from build123d import *

# Parameters (mm, degrees)
SKETCH_1_R          = 14
EXTRUDE_1_DEPTH     = 2.5
SKETCH_2_R          = 1.45
EXTRUDE_2_DEPTH     = 1.5
SKETCH_3_R          = 2.05
CUT_EXTRUDE_1_DEPTH = 21.199009877


with BuildPart() as part:
    # 草图1 → 凸台-拉伸1 (new body)
    with BuildSketch(Plane.XY):
        Circle(SKETCH_1_R)
    extrude(amount=EXTRUDE_1_DEPTH)

    # 草图2 → 凸台-拉伸2 (add)
    with BuildSketch(Plane(origin=(0, 0, 0), x_dir=(-1, 0, 0), z_dir=(0, 0, -1))):
        with Locations(Location((-9.5, 0, 0), (0, 0, 180))):
            Circle(SKETCH_2_R)
        with Locations(Location((0, 8, 0), (0, 0, 180))):
            Circle(SKETCH_2_R)
        with Locations(Location((0, -8, 0), (0, 0, 180))):
            Circle(SKETCH_2_R)
        with Locations(Location((9.5, 0, 0), (0, 0, 180))):
            Circle(SKETCH_2_R)
    extrude(amount=EXTRUDE_2_DEPTH)

    # 草图3 → 切除-拉伸1 (cut, through all)
    with BuildSketch(Plane.XY.offset(2.5)):
        Circle(SKETCH_3_R)
    extrude(amount=-CUT_EXTRUDE_1_DEPTH, mode=Mode.SUBTRACT)

    # 草图4 → 旋转1 (revolve)
    with BuildSketch(Plane(origin=(0, 0, 0), x_dir=(0, 0, -1), z_dir=(1, 0, 0)), mode=Mode.PRIVATE) as revolve_1_sk:
        Polygon((-2.5, 2.05), (-5.70199285, 14), (-2.5, 14), align=None)
    revolve(revolve_1_sk.sketch.rotate(Axis((0, 0, 14.60459965), (0, 0, -1)), 90), axis=Axis((0, 0, 14.60459965), (0, 0, -1)))


solid = part.part
For this review, take the finished solid that the model builds, in its own axes (mm). A direction names the side the tool comes from. Coordinates: 2 decimals unless noted, no trailing zeros. Loops run counter-clockwise (first coordinate to the right, second up) from the corner with the lowest first, then second, coordinate; pieces in that order, holes last. Notation, with made-up numbers: (45, 84.5) -> (94, 84.5) arc R14 ccw to (94, 99.5) -> close; hole circle Ø4 at (-38.75, 80.25). An arc over 180 degrees is marked (long way). Write each question's results on one line, items separated by ' | '.
Q1. Add section C-C, the plane z = 0.5. State the section outline as (x, y) points, then the cut area to 3 significant figures.
Taken from the geometry:
outline: circle Ø28 at (0, 0); hole circle Ø4.1 at (0, 0) | area: 603 mm²
Q2. Machinability: for faces 5 (the conical face through (2.67, -0.84, 2.7)), 6 (the cylindrical face through (-10.95, -0.06, -0.74)), which of the approach directions +Z, -Z, +X, -X, +Y, -Y give a long, thin tool a straight path to every point of the face, cutting with its end or side? Answer none if there is none.
Taken from the geometry:
face 5: +Z | face 6: -Z
Q3. For pin 1 Ø6.5 at (x, y) = (0, 0) entering from -Z; pin 2 Ø4 at (x, y) = (3, -1.5) entering from +Z; pin 3 Ø3 at (y, z) = (6, 4.5) entering from -X, all flat-tipped, find the tip position at first contact; note any pin that passes through.
Taken from the geometry:
pin 1: z = 0 | pin 2: z = 3.39 | pin 3: x = -13.26
Q4. Add section B-B, the plane x = 0. State the section outline as (y, z) points, then the cut area to 3 significant figures.
Taken from the geometry:
outline: (-14, 0) -> (-9.45, 0) -> (-9.45, -1.5) -> (-6.55, -1.5) -> (-6.55, 0) -> (-2.05, 0) -> (-2.05, 2.5) -> (-14, 5.7) -> close; (2.05, 0) -> (6.55, 0) -> (6.55, -1.5) -> (9.45, -1.5) -> (9.45, 0) -> (14, 0) -> (14, 5.7) -> (2.05, 2.5) -> close | area: 107 mm²
Q5. Add section A-A, the plane y = 0. State the section outline as (x, z) points, then the cut area to 3 significant figures.
Taken from the geometry:
outline: (-14, 0) -> (-10.95, 0) -> (-10.95, -1.5) -> (-8.05, -1.5) -> (-8.05, 0) -> (-2.05, 0) -> (-2.05, 2.5) -> (-14, 5.7) -> close; (2.05, 0) -> (8.05, 0) -> (8.05, -1.5) -> (10.95, -1.5) -> (10.95, 0) -> (14, 0) -> (14, 5.7) -> (2.05, 2.5) -> close | area: 107 mm²
Q6. To check wall thickness, follow line 1 along Y through (x, z) = (0, 1.25); line 2 along Z through (x, y) = (2.25, 5.75); line 3 along Z through (x, y) = (1.75, 3.5). State the ranges of each line that lie inside material, in increasing order. Write a range as [from, to].
Taken from the geometry:
line 1: [-14, -2.05], [2.05, 14] | line 2: [0, 3.61] | line 3: [0, 3]
Q7. Add section D-D, the plane z = -1. State the section outline as (x, y) points.
Taken from the geometry:
outline: circle Ø2.9 at (-9.5, 0); circle Ø2.9 at (0, -8); circle Ø2.9 at (0, 8); circle Ø2.9 at (9.5, 0)
Q8. Mouldability with a two-part tool opening along Y and no side actions: class faces 1 (the flat face through (0, -8, -1.5)), 2 (the cylindrical face through (-0.314, 9.416, -0.74)), 3 (the cylindrical face through (8.05, -0.06, -0.74)), 4 (the cylindrical face through (0.669, -6.714, -0.74)) as +Y half, -Y half, draft (parallel to the pull), parting line (faces both ways), or undercut.
Taken from the geometry:
face 1: draft | face 2: undercut | face 3: parting line | face 4: undercut
